Work out the finished part from the listing and answer in its coordinate system (mm). A direction names the side the tool comes from. Coordinates: 2 decimals unless noted, no trailing zeros. Order: outer loops, then holes, each group sorted by start corner. A loop starts at its lowest first (then second) coordinate and runs counter-clockwise, first axis right, second up. Notation, with made-up numbers: M 89,70 L 104,70 A15 ccw 104,90 Z; hole C 83,12 d8. An arc over 180 degrees is marked long. Use a Markdown table: item, result.
from build123d import *

# Parameters (mm, degrees)
F0_W           = 90.678
F0_H           = 217.4875
F1_DEPTH       = 17.145
F3_D           = 4.826
F3_CSINK_D     = 9.398
F3_CSINK_ANGLE = 84
F2_R           = 17.4625
F2_R_2         = 6.35
F2_R_3         = 2.54
F4_DEPTH       = 25.4
F5_W           = 77.978
F5_H           = 204.7875
F5_R           = 2.413
F5_R_2         = 17.4625
F5_R_3         = 6.35
F5_R_4         = 2.54
F6_DEPTH       = 12.065
F7_D           = 4.826
F7_CSINK_D     = 9.398
F7_CSINK_ANGLE = 84
F8_W           = 90.678
F8_H           = 81.915
F9_DEPTH       = 17.145
F10_W          = 63.754
F10_H          = 59.69
F11_DEPTH      = 17.146
F12_DEPTH      = 1.524
F13_W          = 9.525
F13_H          = 9.525
F13_R          = 2.54
F14_DEPTH      = 1.524
F15_R          = 5.08
F16_R          = 15.24
F17_R          = 1.5875


with BuildPart() as f1:
    # F0 (on Front) → F1 (new body)
    with BuildSketch(Plane.XZ):
        with Locations((45.339, 108.74375)):
            Rectangle(F0_W, F0_H)
    extrude(amount=F1_DEPTH)

    # F3 (through all)
    with Locations(Plane.XZ.offset(17.145)):
        with Locations((45.339, 22.86)):
            CounterSinkHole(F3_D / 2, F3_CSINK_D / 2, counter_sink_angle=F3_CSINK_ANGLE)

    # F2 (on face) → F4 (cut)
    with BuildSketch(Plane.XZ.offset(17.145)):
        with Locations((45.339, 63.5)):
            Circle(F2_R)
        with Locations((45.339, 160.3375)):
            Circle(F2_R_2)
        with Locations((33.147, 163.5125)):
            Circle(F2_R_3)
        with Locations((57.531, 163.5125)):
            Circle(F2_R_3)
    extrude(amount=-F4_DEPTH, mode=Mode.SUBTRACT)

    # F5 (on face) → F6 (cut)
    with BuildSketch(Plane(origin=(0, 0, 0), x_dir=(-1, 0, 0), z_dir=(0, 1, 0))):
        with Locations((-45.339, 108.74375)):
            Rectangle(F5_W, F5_H)
        with Locations((-45.339, 22.86)):
            Circle(F5_R, mode=Mode.SUBTRACT)
        with Locations((-45.339, 63.5)):
            Circle(F5_R_2, mode=Mode.SUBTRACT)
        with Locations((-45.339, 160.3375)):
            Circle(F5_R_3, mode=Mode.SUBTRACT)
        with Locations((-57.531, 163.5125)):
            Circle(F5_R_4, mode=Mode.SUBTRACT)
        with Locations((-33.147, 163.5125)):
            Circle(F5_R_4, mode=Mode.SUBTRACT)
    extrude(amount=-F6_DEPTH, mode=Mode.SUBTRACT)

    # F7 (through all)
    with Locations(Plane.XZ.offset(17.145)):
        with Locations((45.339, 143.3195)):
            CounterSinkHole(F7_D / 2, F7_CSINK_D / 2, counter_sink_angle=F7_CSINK_ANGLE)

    # F8 (on Front) → F9 (join, through all)
    with BuildSketch(Plane.XZ):
        with Locations((45.339, 258.445)):
            Rectangle(F8_W, F8_H)
    extrude(amount=F9_DEPTH)

    # F10 (on face) → F11 (cut, through all)
    with BuildSketch(Plane(origin=(0, 0, 0), x_dir=(-1, 0, 0), z_dir=(0, 1, 0))):
        with Locations((-45.339, 260.6675)):
            Rectangle(F10_W, F10_H)
    extrude(amount=-F11_DEPTH, mode=Mode.SUBTRACT)

    # F2 (on face) → F12 (cut)
    with BuildSketch(Plane.XZ.offset(17.145)):
        with BuildLine():
            ThreePointArc((54.4352503264, 150.8125), (61.8498032005, 157.8882238651), (64.5795, 167.767))
            ThreePointArc((64.5795, 167.767), (35.4602238651, 184.2778032005), (36.2427496736, 150.8125))
            Line((36.2427496736, 150.8125), (54.4352503264, 150.8125))
        make_face()
        with Locations((45.339, 160.3375)):
            Circle(F2_R_2, mode=Mode.SUBTRACT)
        with Locations((33.147, 163.5125)):
            Circle(F2_R_3, mode=Mode.SUBTRACT)
        with Locations((57.531, 163.5125)):
            Circle(F2_R_3, mode=Mode.SUBTRACT)
    extrude(amount=-F12_DEPTH, mode=Mode.SUBTRACT)

    # F13 (on face) → F14 (cut)
    with BuildSketch(Plane(origin=(0, -12.065, 0), x_dir=(-1, 0, 0), z_dir=(0, 1, 0))):
        with Locations((-57.531, 163.5125)):
            Rectangle(F13_W, F13_H)
        with Locations((-57.531, 163.5125)):
            Circle(F13_R, mode=Mode.SUBTRACT)
        with Locations((-33.147, 163.5125)):
            Rectangle(F13_W, F13_H)
        with Locations((-33.147, 163.5125)):
            Circle(F13_R, mode=Mode.SUBTRACT)
    extrude(amount=-F14_DEPTH, mode=Mode.SUBTRACT)

    # F15
    f15_edges = [f1.edges().sort_by_distance(p)[0] for p in [
        (84.328, -6.0325, 211.1375),
        (6.35, -6.0325, 211.1375),
        (6.35, -6.0325, 6.35),
        (84.328, -6.0325, 6.35),
    ]]
    fillet(f15_edges, radius=F15_R)

    # F16
    f16_edges = [f1.edges().sort_by_distance(p)[0] for p in [
        (90.678, -8.5725, 0),
        (0, -8.5725, 0),
        (0, -8.5725, 299.4025),
        (90.678, -8.5725, 299.4025),
    ]]
    fillet(f16_edges, radius=F16_R)

    # F17
    f17_edges = [f1.edges().sort_by_distance(p)[0] for p in [
        (0, -17.145, 149.70125),
        (45.339, -17.145, 0),
        (4.463693, -17.145, 4.463693),
        (86.214307, -17.145, 4.463693),
        (90.678, -17.145, 149.70125),
        (4.463693, -17.145, 294.938807),
        (86.214307, -17.145, 294.938807),
        (45.339, -17.145, 299.4025),
    ]]
    fillet(f17_edges, radius=F17_R)


solid = f1.part
1. For a pull along X with two mould halves and no side action, classify faces 4 (the face through (86.095, -7.888, 295.057)), 5 (the face through (7.8, -6.12, 209.61)), 6 (the face through (0, -8, 148)), 7 (the face through (45, -8, 0)) as +X half, -X half, draft (parallel to the pull), parting line (faces both ways), or undercut.
Answers below:
| item | result |
|---|---|
| face 4 | +X half |
| face 5 | undercut |
| face 6 | -X half |
| face 7 | draft |
2. For faces 1 (the face through (44.17, -14.73, 141.08)), 2 (the face through (77.216, -8, 260)), 3 (the face through (7.799, -6.117, 7.878)), determine the directions among +Z, -Z, +X, -X, +Y, -Y from which every point of the face is accessible in a straight line to the end or side of a thin tool.
Answers below:
| item | result |
|---|---|
| face 1 | -Y |
| face 2 | +Y, -Y |
| face 3 | +Y |
3. Find the intervals of material crossed by probe 1 along Z at (x, y) = (28, -4.25); probe 2 along X at (y, z) = (-2.25, 233); probe 3 along X at (y, z) = (-12.7, 22.86), in increasing order.
Answers below:
| item | result |
|---|---|
| probe 1 | 0 to 6.35, 211.14 to 230.82, 290.51 to 299.4 |
| probe 2 | 0 to 13.46, 77.22 to 90.68 |
| probe 3 | 0 to 42.93, 47.75 to 90.68 |
4. Section C-C on y = -4.5 is taken. Determine the outline of the cut face in (x, z), then the cut area to 3 significant figures.
Answers below:
| item | result |
|---|---|
| outline | M 0,15.24 A15.24 ccw 15.24,0 L 75.44,0 A15.24 ccw 90.68,15.24 L 90.68,284.16 A15.24 ccw 75.44,299.4 L 15.24,299.4 A15.24 ccw 0,284.16 Z; hole M 6.35,11.43 A5.08 ccw 11.43,6.35 L 79.25,6.35 A5.08 ccw 84.33,11.43 L 84.33,206.06 A5.08 ccw 79.25,211.14 L 11.43,211.14 A5.08 ccw 6.35,206.06 Z; hole M 13.46,230.82 L 77.22,230.82 L 77.22,290.51 L 13.46,290.51 Z |
| area | 7,200 mm² |
5. A flat-ended cylindrical pin translates along its axis: P1, Ø23, axis at x = 45.339, z = 167.767, coming from the +Y side (3 decimals). Find the tip coordinate at first contact, or state that the pin passes through.
Answers below:
| item | result |
|---|---|
| P1 | y = -12.065 |
